Here's how the part is built. I have some questions about the finished solid (model axes, mm). A direction names the side the tool comes from. Round coordinates to 2 decimals unless told otherwise and drop trailing zeros. Order: outer loops, then holes, each group sorted by start corner. A loop starts at its lowest first (then second) coordinate and runs counter-clockwise, first axis right, second up. Notation, with made-up numbers: (-25, 13) -> (3, 13) arc R26 ccw to (3, 31) -> close; hole circle Ø2 at (10.5, -20.5). An arc over 180 degrees is marked (long way). Use a Markdown table: item, result. Add a question column.
from build123d import *

# Parameters (mm, degrees)
F0_W     = 100
F0_H     = 45
F0_R     = 2
F0_R_2   = 3
F0_R_3   = 4
F0_W_2   = 6.83609
F0_H_2   = 36.256011
F0_R_4   = 7
F0_R_5   = 2.5
F0_R_6   = 6
F0_W_3   = 14.703342
F0_H_3   = 35.687724
F1_DEPTH = 20
F2_R     = 2.15
F3_DEPTH = 50
F4_R     = 4
F5_DEPTH = 40


with BuildPart() as f1:
    # F0 (on Front) → F1 (new body)
    with BuildSketch(Plane.XZ):
        with Locations((-3.569908, 42.308319)):
            Rectangle(F0_W, F0_H)
        with Locations((-36.130425, 30.930979)):
            Circle(F0_R, mode=Mode.SUBTRACT)
        with Locations((-24.125798, 30.930979)):
            Circle(F0_R_2, mode=Mode.SUBTRACT)
        with Locations((-15.455791, 30.930979)):
            Circle(F0_R, mode=Mode.SUBTRACT)
        with Locations((-8.11963, 30.930979)):
            Circle(F0_R_3, mode=Mode.SUBTRACT)
        with Locations((-45.552673, 42.154359)):
            Rectangle(F0_W_2, F0_H_2, mode=Mode.SUBTRACT)
        with Locations((7.382729, 30.930979)):
            Circle(F0_R_4, mode=Mode.SUBTRACT)
        with Locations((-36.130425, 42.308319)):
            Circle(F0_R, mode=Mode.SUBTRACT)
        with Locations((-24.125798, 42.308319)):
            Circle(F0_R_5, mode=Mode.SUBTRACT)
        with Locations((-15.455791, 42.308319)):
            Circle(F0_R, mode=Mode.SUBTRACT)
        with Locations((-8.11963, 42.308319)):
            Circle(F0_R_3, mode=Mode.SUBTRACT)
        with Locations((-36.130425, 53.91388)):
            Circle(F0_R, mode=Mode.SUBTRACT)
        with Locations((-24.125798, 53.91388)):
            Circle(F0_R_5, mode=Mode.SUBTRACT)
        with Locations((-15.455791, 53.91388)):
            Circle(F0_R, mode=Mode.SUBTRACT)
        with Locations((-8.11963, 53.91388)):
            Circle(F0_R_3, mode=Mode.SUBTRACT)
        with Locations((18.517302, 42.308319)):
            Circle(F0_R_6, mode=Mode.SUBTRACT)
        with Locations((35.576041, 42.493804)):
            Rectangle(F0_W_3, F0_H_3, mode=Mode.SUBTRACT)
        with Locations((7.382729, 53.91388)):
            Circle(F0_R_4, mode=Mode.SUBTRACT)
    extrude(amount=F1_DEPTH)

    # F2 (on face) → F3 (cut)
    with BuildSketch(Plane(origin=(0, 0, 19.808319), x_dir=(1, 0, 0), z_dir=(0, 0, -1))):
        with Locations((21.430092, 10)):
            Circle(F2_R)
        with Locations((-28.569908, 10)):
            Circle(F2_R)
    extrude(amount=-F3_DEPTH, mode=Mode.SUBTRACT)

    # F4 (on face) → F5 (cut)
    with BuildSketch(Plane(origin=(0, 0, 19.808319), x_dir=(1, 0, 0), z_dir=(0, 0, -1))):
        with Locations((-28.569908, 10)):
            Circle(F4_R)
        with Locations((21.430092, 10)):
            Circle(F4_R)
    extrude(amount=-F5_DEPTH, mode=Mode.SUBTRACT)


solid = f1.part
(1) I want a section at A-A on x = -43.5. List the corners of the cut face in (y, z) for me, and give its area (3 significant figures).
(2) If we mould it in two halves opening along Y, with no side actions, what happens to faces 1 (the cylindrical face through (-32.566, -10.176, 39.528)), 2 (the cylindrical face through (-8.99, -9.86, 50.01))? For each: pulls with the +Y half, pulls with the -Y half, needs draft (parallel to the pull), parting line crosses it, or undercut.
(3) I want a section at B-B on y = -15.25. State how many separate pieces and enclosed holes the cut face has, and give its area (3 significant figures).
(4) On a 3-axis mill with a long thin cutter (end or side, diameter ignored), from which of +Z, -Z, +X, -X, +Y, -Y can I reach the whole of each face in a straight line? I mean faces 3 (the flat face through (46.43, -10, 42)), 4 (the flat face through (-46, -10, 60.282)), 5 (the flat face through (-27, -8, 59.808)). Say none if no direction works.
(5) I want a section at C-C on x = 22. List the corners of the cut face in (y, z) for me, and give its area (3 significant figures).
(6) Please list where these lines run through material, in increasing order: probe 1 along Z at (x, y) = (7.5, -7.5); probe 2 along X at (y, z) = (-8, 45.5); probe 3 along Z at (x, y) = (-36.5, -8.5). Write a range as from..to.
(7) I'm going to push flat-ended pins straight in: P1, Ø3.5, axis at x = -15.46, z = 30.93, coming from the +Y side; P2, Ø7, axis at x = 21.43, y = -10, coming from the -Z side. Where does each tip first touch, or does it pass through?
Output:
| question | item | result |
|---|---|---|
| 1 | outline | (-20, 19.81) -> (0, 19.81) -> (0, 24.03) -> (-20, 24.03) -> close; (-20, 60.28) -> (0, 60.28) -> (0, 64.81) -> (-20, 64.81) -> close |
| 1 | area | 175 mm² |
| 2 | face 1 | undercut |
| 2 | face 2 | needs draft |
| 3 | separate pieces | 1 |
| 3 | enclosed holes | 17 |
| 3 | area | 3,010 mm² |
| 4 | face 3 | +Z, -Z, +X, +Y, -Y |
| 4 | face 4 | +Y, -Y |
| 4 | face 5 | -Z |
| 5 | outline | (-20, 19.81) -> (-13.96, 19.81) -> (-13.96, 37.42) -> (-20, 37.42) -> close; (-20, 47.19) -> (-13.96, 47.19) -> (-13.96, 59.81) -> (-12.07, 59.81) -> (-12.07, 64.81) -> (-20, 64.81) -> close; (-7.93, 59.81) -> (-6.04, 59.81) -> (-6.04, 47.19) -> (0, 47.19) -> (0, 64.81) -> (-7.93, 64.81) -> close; (-6.04, 19.81) -> (0, 19.81) -> (0, 37.42) -> (-6.04, 37.42) -> close |
| 5 | area | 444 mm² |
| 6 | probe 1 | 19.81..23.93, 37.93..46.91, 60.91..64.81 |
| 6 | probe 2 | -53.57..-48.97, -42.13..-32.03, -25.11..-10.53, -5.71..13.44, 24.89..28.22, 42.93..46.43 |
| 6 | probe 3 | 19.81..28.97, 32.9..40.34, 44.27..51.95, 55.88..64.81 |
| 7 | P1 | through |
| 7 | P2 | z = 59.81 |
